```python
from build123d import *

# Parameters (mm, degrees)
Y_KSEKLIK_EKSTR_ZYON6_DEPTH      = 15
Y_KSEKLIK_EKSTR_ZYON6_DEPTH_BACK = 10
Y_KSEKLIK_EKSTR_ZYON7_DEPTH      = 5
Y_KSEKLIK_EKSTR_ZYON7_DEPTH_BACK = 5


with BuildPart() as part:
    # izim2 → Y_kseklik-Ekstr_zyon6 (new, two sides: drawn at the far end of the back side and taken through both)
    with BuildSketch(Plane.XY.offset(-Y_KSEKLIK_EKSTR_ZYON6_DEPTH_BACK)):
        with BuildLine():
            ThreePointArc((-4.224237601, 35.120848822), (-6.602172627, 28.000835961), (-7.4071606, 20.537515488))
            Line((-7.4071606, 20.537515488), (7.5928394, 20.537515488))
            ThreePointArc((7.5928394, 20.537515488), (27.5928394, 40.537515488), (47.5928394, 20.537515488))
            Line((47.5928394, 20.537515488), (62.5928394, 20.537515488))
            ThreePointArc((62.5928394, 20.537515488), (35.056159873, 54.732527515), (-4.224237601, 35.120848822))
        make_face()
        with BuildLine():
            Line((7.5928394, 20.537515488), (-7.4071606, 20.537515488))
            ThreePointArc((-7.4071606, 20.537515488), (23.973490262, -14.274843119), (61.844285789, 13.337625196))
            ThreePointArc((61.844285789, 13.337625196), (62.405198007, 16.918166351), (62.5928394, 20.537515488))
            Line((62.5928394, 20.537515488), (47.5928394, 20.537515488))
            ThreePointArc((47.5928394, 20.537515488), (27.5928394, 0.537515488), (7.5928394, 20.537515488))
        make_face()
    extrude(amount=Y_KSEKLIK_EKSTR_ZYON6_DEPTH + Y_KSEKLIK_EKSTR_ZYON6_DEPTH_BACK)

    # izim2_9 → Y_kseklik-Ekstr_zyon7 (add, two sides: drawn at the far end of the back side and taken through both)
    with BuildSketch(Plane.XY.offset(-Y_KSEKLIK_EKSTR_ZYON7_DEPTH_BACK)):
        with BuildLine():
            ThreePointArc((61.844285789, 13.337625196), (16.633425799, -12.702389047), (-4.224237601, 35.120848822))
            ThreePointArc((-4.224237601, 35.120848822), (-13.449178052, 24.4968802), (-26.950721174, 20.537515488))
            Line((-26.950721174, 20.537515488), (-38.44931098, 20.537515488))
            ThreePointArc((-38.44931098, 20.537515488), (-51.701711944, 15.516629904), (-58.300234012, 2.974902357))
            Line((-58.300234012, 2.974902357), (-60.95730449, -18.665200093))
            ThreePointArc((-60.95730449, -18.665200093), (-58.156545185, -24.500240081), (-51.684983771, -24.396138183))
            Line((-51.684983771, -24.396138183), (-15.993696643, -4.166774273))
            ThreePointArc((-15.993696643, -4.166774273), (-15.929312008, -4.130595361), (-15.864661939, -4.094892934))
            ThreePointArc((-15.864661939, -4.094892934), (-5.960873253, -4.265931617), (-1.062781275, -12.875401956))
            ThreePointArc((-1.062781275, -12.875401956), (27.996215902, -61.128273793), (70.546183821, -98.037150605))
            Line((70.546183821, -98.037150605), (98.484313975, -102.963396742))
            ThreePointArc((98.484313975, -102.963396742), (102.831933538, -100.653703951), (101.646021849, -95.875619594))
            ThreePointArc((101.646021849, -95.875619594), (66.141131912, -46.955735677), (61.844285789, 13.337625196))
        make_face()
    extrude(amount=Y_KSEKLIK_EKSTR_ZYON7_DEPTH + Y_KSEKLIK_EKSTR_ZYON7_DEPTH_BACK)


solid = part.part
```
Model file for the job. Use its own axes, mm. A direction names the side the tool comes from. Coordinates: 2 decimals unless noted, no trailing zeros. Write each loop counter-clockwise with the first axis right and the second up, starting at its lowest first coordinate (ties: lowest second). Pieces come first, ordered by that corner, then holes. Notation, with made-up numbers: (9, 25.5) - (54, 25.5) arc R12 cw to (54, 39.5) - close; hole circle Ø9 at (-37, 71.25). An arc over 180 degrees is marked (long way). One line per item, written item: value. Start each with the question number.
1. Tool access for faces 1 (the flat face through (-34.089, -14.423, -0.07)), 2 (the flat face through (-33, 20.538, 0)), 3 (the cylindrical face through (66.438, -47.76, -0.07)): list every direction of +Z, -Z, +X, -X, +Y, -Y with a clear straight run to the whole face (end or side of a thin tool).
2. Mould opens along Y. For faces 4 (the flat face through (21, -29, -5)), 5 (the cylindrical face through (46.068, 28.198, 2.325)), 6 (the flat face through (84.32, -100.466, -0.07)) say: released by +Y, released by -Y, zero draft, split by the parting line, or undercut.
3. Probe line 1 (Y direction, x = 27.5, z = 5.75); line 2 (Z direction, x = -31.5, y = -5.5); line 3 (Y direction, x = 24, z = 8.25). List the from-to ranges inside material, lowest first. Write a range as from..to.
4. Flat gauge pins, fed straight in: pin 1 (12 mm diameter, centred on y = 0, z = 0, fed in from +X); pin 2 (1 mm diameter, centred on y = -14, z = -4.5, fed in from -X); pin 3 (12 mm diameter, centred on y = -85.5, z = -2.5, fed in from -X). Where does each tip first touch, or does it go through?
5. Slice it at D-D (y = 28). Write the cut outline in (x, z), plus the area to 3 significant figures.
6. Slice it at C-C (x = 21.5). Write the cut outline in (y, z).
7. Slice it at A-A (z = 2). Write the cut outline in (x, y).
8. Slice it at B-B (y = -7). Write the cut outline in (x, z) (3 decimals), plus the area to 3 significant figures.
Answers below:
1. face 1: +Z, -Z, -Y
1. face 2: +Z, -Z, -X, +Y
1. face 3: +Z, -Z, +X
2. face 4: zero draft
2. face 5: undercut
2. face 6: released by -Y
3. line 1: y = -14.46..0.54, 40.54..55.54
3. line 2: z = -5..5
3. line 3: y = -14.28..0.86, 40.21..55.35
4. pin 1: stops at x = 60.56
4. pin 2: stops at x = -60.45
4. pin 3: stops at x = 45.82
5. outline: (-9.13, -5) - (-6.6, -5) - (-6.6, -10) - (9.04, -10) - (9.04, 15) - (-6.6, 15) - (-6.6, 5) - (-9.13, 5) - close; (46.15, -10) - (61.79, -10) - (61.79, 15) - (46.15, 15) - close
5. area: 807 mm^2
6. outline: (-52.93, -5) - (-13.93, -5) - (-13.93, -10) - (1.49, -10) - (1.49, 15) - (-13.93, 15) - (-13.93, 5) - (-52.93, 5) - close; (39.59, -10) - (55, -10) - (55, 15) - (39.59, 15) - close
7. outline: (-60.96, -18.67) arc R6 ccw to (-51.68, -24.4) - (-15.99, -4.17) arc R10 cw to (-15.86, -4.09) arc R10 cw to (-1.06, -12.88) arc R180 ccw to (70.55, -98.04) - (98.48, -102.96) arc R4 ccw to (101.65, -95.88) arc R110 cw to (61.84, 13.34) arc R35 ccw to (-4.22, 35.12) arc R25 cw to (-26.95, 20.54) - (-38.45, 20.54) arc R20 ccw to (-58.3, 2.97) - close; hole circle Ø40 at (27.59, 20.54)
8. outline: (-59.525, -5) - (-20.992, -5) - (-20.992, 5) - (-59.525, 5) - close; (-2.964, -5) - (5.99, -5) - (5.99, -10) - (49.196, -10) - (49.196, -5) - (59.516, -5) - (59.516, 5) - (49.196, 5) - (49.196, 15) - (5.99, 15) - (5.99, 5) - (-2.964, 5) - close
8. area: 1,660 mm^2
